Check sheet for the modelled part. Datum: model origin and axes. Units: mm. A direction names the side the tool comes from. Round coordinates to 2 decimals unless told otherwise and drop trailing zeros. Loops run counter-clockwise (first coordinate to the right, second up) from the corner with the lowest first, then second, coordinate; pieces in that order, holes last. Notation, with made-up numbers: (17.5, -1) -> (54.5, -1) arc R23 cw to (54.5, 18) -> close; hole circle Ø5 at (15, 34). An arc over 180 degrees is marked (long way). One line per question, with ' | ' between items.
```python
from build123d import *

# Parameters (mm, degrees)
F1_DEPTH  = 125
F2_R      = 1.85
F3_DEPTH  = 4
F5_DEPTH  = 3
F7_R      = 6
F8_DEPTH  = 25
F10_R     = 6
F11_DEPTH = 25


with BuildPart() as f1:
    # F0 (on Front) → F1 (new body)
    with BuildSketch(Plane.XZ):
        Polygon((27.4241377865, 47.5), (-27.4241377865, 47.5), (-23.9600361714, 41.5), (23.9600361714, 41.5), align=None)
    extrude(amount=F1_DEPTH)

    # F2 (on face) → F3 (cut)
    with BuildSketch(Plane(origin=(0, 0, 41.5), x_dir=(1, 0, 0), z_dir=(0, 0, -1))):
        with BuildLine():
            ThreePointArc((-13.8300180857, 120), (-11.9800180857, 118.15), (-10.1300180857, 120))
            Line((-10.1300180857, 120), (-13.8300180857, 120))
        make_face()
        with BuildLine():
            Line((-13.8300180857, 120), (-10.1300180857, 120))
            ThreePointArc((-10.1300180857, 120), (-11.9800180857, 121.85), (-13.8300180857, 120))
        make_face()
        with Locations((11.9800180857, 120)):
            Circle(F2_R)
        with BuildLine():
            ThreePointArc((-13.8300180857, 23), (-11.9800180857, 21.15), (-10.1300180857, 23))
            Line((-10.1300180857, 23), (-13.8300180857, 23))
        make_face()
        with BuildLine():
            Line((-13.8300180857, 23), (-10.1300180857, 23))
            ThreePointArc((-10.1300180857, 23), (-11.9800180857, 24.85), (-13.8300180857, 23))
        make_face()
        with Locations((11.9800180857, 23)):
            Circle(F2_R)
    extrude(amount=-F3_DEPTH, mode=Mode.SUBTRACT)

    # F4 (on face) → F5 (join)
    with BuildSketch(Plane.XY.offset(47.5)):
        Polygon((0.5340071506, -61.535328541), (-0.4659928494, -62.1126788102), (-0.4659928494, -65.5259274643), (-0.4659928494, -66.6806280026), (-0.4659928494, -67.4806280026), (-0.4659928494, -68.635328541), (-0.4659928494, -69.3806280026), (1.5340071506, -69.3806280026), (1.5340071506, -68.635328541), (1.5340071506, -67.4806280026), (1.5340071506, -66.6806280026), (1.5340071506, -65.5259274643), (1.5340071506, -62.1126788102), align=None)
        Polygon((2.900031855, -68.2693027335), (1.5340071506, -67.4806280026), (1.5340071506, -68.635328541), (2.4000325544, -69.135328541), align=None)
        Polygon((4.132083362, -67.0259274643), (1.5340071506, -65.5259274643), (1.5340071506, -66.6806280026), (3.6320840614, -67.8919532719), align=None)
        Polygon((-0.4659928494, -68.635328541), (-0.4659928494, -67.4806280026), (-1.8520648707, -68.2808770573), (-1.3320182531, -69.135328541), align=None)
        Polygon((-0.4659928494, -66.6806280026), (-0.4659928494, -65.5259274643), (-3.0640690607, -67.0259274643), (-2.5440224431, -67.880378948), align=None)
        Polygon((-3.4219535926, -66.819303541), (-3.4219535926, -63.819303541), (-4.4219535926, -64.3966538102), (-4.4219535926, -66.819303541), align=None)
        Polygon((-5.1147739156, -66.5781745553), (-5.1147739156, -64.7966538102), (-6.1147739156, -65.3740040794), (-6.1147739156, -66.5781745553), align=None)
        Polygon((-7.1147739156, -63.6419532718), (-6.1147739156, -63.0646030026), (-7.6576161382, -62.1738426302), (-8.1576161382, -63.039868034), align=None)
        Polygon((-5.4219535926, -62.6646030026), (-4.4219535926, -62.0872527334), (-7.0200298039, -60.5872527335), (-7.5200298039, -61.4532781373), align=None)
        Polygon((-4.4219535925, -58.6740032718), (-5.4219535925, -58.0966530026), (-7.5200298039, -59.307977868), (-7.0200298039, -60.1740032718), align=None)
        Polygon((-8.1576161382, -57.7213879713), (-7.6576161382, -58.5874133751), (-6.1147739156, -57.6966530026), (-7.1147739156, -57.1193027334), align=None)
        Polygon((-6.1147739156, -54.18308145), (-6.1147739156, -55.3872519259), (-5.1147739156, -55.964602195), (-5.1147739156, -54.18308145), align=None)
        Polygon((-4.4219535926, -53.9419524643), (-4.4219535926, -56.3646021951), (-3.4219535925, -56.9419524642), (-3.4219535926, -53.9419524643), align=None)
        Polygon((-3.0640690607, -53.735328541), (-0.4659928494, -55.235328541), (-0.4659928494, -54.0806280026), (-2.5440224431, -52.8808770573), align=None)
        Polygon((-1.8520648707, -52.480378948), (-0.4659928494, -53.2806280026), (-0.4659928494, -52.1259274643), (-1.3320182531, -51.6259274643), align=None)
        Polygon((1.5340071506, -52.1259274643), (1.5340071506, -53.2806280026), (2.900031855, -52.4919532718), (2.4000325544, -51.6259274643), align=None)
        Polygon((1.5340071506, -54.0806280026), (1.5340071506, -55.235328541), (4.132083362, -53.735328541), (3.6320840614, -52.8693027334), align=None)
        Polygon((4.4899678938, -53.9419524643), (4.4899678938, -56.9419524643), (5.4899678938, -56.3646021951), (5.4899678938, -53.9419524643), align=None)
        Polygon((6.1827882169, -54.18308145), (6.1827882169, -55.9646021951), (7.1827882169, -55.3872519259), (7.1827882169, -54.18308145), align=None)
        Polygon((8.1827882169, -57.1193027334), (7.1827882169, -57.6966530026), (8.7256304395, -58.5874133751), (9.2256304395, -57.7213879713), align=None)
        Polygon((6.4899678939, -58.0966530026), (5.4899678939, -58.6740032718), (8.0880441052, -60.1740032718), (8.5880441052, -59.307977868), align=None)
        Polygon((8.0880441052, -60.5872527335), (5.4899678939, -62.0872527335), (6.4899678939, -62.6646030027), (8.5880441052, -61.4532781373), align=None)
        Polygon((8.7256304395, -62.1738426302), (7.1827882169, -63.0646030027), (8.1827882169, -63.6419532719), (9.2256304395, -63.039868034), align=None)
        Polygon((7.1827882169, -65.3740040794), (6.1827882169, -64.7966538102), (6.1827882169, -66.5781745553), (7.1827882169, -66.5781745553), align=None)
        Polygon((2.5340071506, -60.3806280026), (1.5340071506, -60.9579782718), (1.5340071506, -62.1126788102), (4.4899678938, -63.819303541), (5.4899678938, -64.3966538102), (6.1827882169, -64.7966538102), (7.1827882169, -65.3740040794), (7.8282364841, -65.7466538103), (8.8282350853, -64.0146021951), (8.1827882169, -63.6419532719), (7.1827882169, -63.0646030027), (6.4899678939, -62.6646030027), (5.4899678939, -62.0872527335), align=None)
        Polygon((-0.4659928494, -60.9579782718), (-1.4659928493, -60.3806280026), (-4.4219535926, -62.0872527334), (-5.4219535926, -62.6646030026), (-6.1147739156, -63.0646030026), (-7.1147739156, -63.6419532718), (-7.7602214834, -64.0146025988), (-6.7602214834, -65.7466534064), (-6.1147739156, -65.3740040794), (-5.1147739156, -64.7966538102), (-4.4219535926, -64.3966538102), (-3.4219535926, -63.819303541), (-0.4659928494, -62.1126788102), align=None)
        Polygon((-7.1147739156, -57.1193027334), (-6.1147739156, -57.6966530026), (-5.4219535925, -58.0966530026), (-4.4219535925, -58.6740032718), (-1.4659928493, -60.3806280026), (-0.4659928494, -59.8032777334), (-0.4659928494, -58.648577195), (-3.4219535925, -56.9419524642), (-4.4219535925, -56.364602195), (-5.1147739156, -55.964602195), (-6.1147739156, -55.3872519258), (-6.7602221828, -55.014602195), (-7.760220784, -56.7466538101), align=None)
        Polygon((1.5340071506, -58.648577195), (1.5340071506, -59.8032777334), (2.5340071506, -60.3806280026), (5.4899678939, -58.6740032718), (6.4899678939, -58.0966530026), (7.1827882169, -57.6966530026), (8.1827882169, -57.1193027334), (8.8282357847, -56.7466534064), (7.8282357847, -55.0146025988), (7.1827882169, -55.3872519259), (6.1827882169, -55.9646021951), (5.4899678938, -56.3646021951), (4.4899678938, -56.9419524643), align=None)
        Polygon((-0.4659928494, -55.235328541), (-0.4659928494, -58.648577195), (0.5340071506, -59.2259274642), (1.5340071506, -58.648577195), (1.5340071506, -55.235328541), (1.5340071506, -54.0806280026), (1.5340071506, -53.2806280026), (1.5340071506, -52.1259274643), (1.5340071506, -51.3806280026), (-0.4659928494, -51.3806280026), (-0.4659928494, -52.1259274643), (-0.4659928494, -53.2806280026), (-0.4659928494, -54.0806280026), align=None)
        Polygon((5.4899678938, -64.3966538102), (4.4899678938, -63.819303541), (4.4899678938, -66.819303541), (5.4899678938, -66.819303541), align=None)
        Polygon((0.5340071506, -61.535328541), (-0.4659928494, -60.9579782718), (-0.4659928494, -62.1126788102), align=None)
        Polygon((1.5340071506, -60.9579782718), (0.5340071506, -61.535328541), (1.5340071506, -62.1126788102), align=None)
        Polygon((2.5340071506, -60.3806280026), (1.5340071506, -59.8032777334), (1.5340071506, -60.9579782718), align=None)
        Polygon((1.5340071506, -58.648577195), (0.5340071506, -59.2259274642), (1.5340071506, -59.8032777334), align=None)
        Polygon((0.5340071506, -59.2259274642), (-0.4659928494, -59.8032777334), (-0.4659928494, -60.9579782718), (0.5340071506, -61.535328541), (1.5340071506, -60.9579782718), (1.5340071506, -59.8032777334), align=None)
        Polygon((-0.4659928494, -59.8032777334), (-1.4659928493, -60.3806280026), (-0.4659928494, -60.9579782718), align=None)
        Polygon((-0.4659928494, -58.648577195), (-0.4659928494, -59.8032777334), (0.5340071506, -59.2259274642), align=None)
    extrude(amount=F5_DEPTH)

    # F7 (on face) → F8 (cut)
    with BuildSketch(Plane(origin=(-23.9600361714, 0, 41.5), x_dir=(0.8660254038, 0, 0.5), z_dir=(0.5, 0, -0.8660254038))):
        with Locations((0, 62.5)):
            Circle(F7_R)
    extrude(amount=F8_DEPTH, mode=Mode.SUBTRACT)

    # F10 (on face) → F11 (cut)
    with BuildSketch(Plane(origin=(23.9600361714, 0, 41.5), x_dir=(0.8660254038, 0, -0.5), z_dir=(0.5, 0, 0.8660254038))):
        with Locations((0, -62.5)):
            Circle(F10_R)
    extrude(amount=-F11_DEPTH, mode=Mode.SUBTRACT)


solid = f1.part
```
(1) Sectioned sample at B-B, the plane z = 43. Count the separate pieces of the cut face and the enclosed holes in it, and give its area (3 significant figures).
Answer:
separate pieces: 1 | enclosed holes: 6 | area: 6,110 mm2
(2) Scan lines: probe 1 along Z at (x, y) = (-11, -36); probe 2 along Y at (x, z) = (-6.5, 48.5); probe 3 along Y at (x, z) = (11, 42). Record each from-to range of solid material in increasing order.
Answer:
probe 1: z = 41.5 to 47.5 | probe 2: y = -65.6 to -62.84, -62.04 to -60.89, -59.87 to -58.72, -57.92 to -55.16 | probe 3: y = -125 to -121.57, -118.43 to -24.57, -21.43 to 0
(3) Mould release check, pull along Y, two halves, no side actions. Record for faces 5 (the face through (0, -125, 45)), 6 (the face through (6.807, -61.327, 48.979)), 7 (the face through (0, -60, 50.5)): +Y half, -Y half, draft (parallel to the pull), parting line (faces both ways), or undercut.
Answer:
face 5: -Y half | face 6: undercut | face 7: draft
(4) Set-up check for faces 1 (the face through (11.739, -121.834, 43.472)), 2 (the face through (25.67, -61.62, 44.46)), 3 (the face through (-3.422, -65, 49)), 4 (the face through (-1.747, -66.265, 48.979)): record each of +Z, -Z, +X, -X, +Y, -Y from which the full face is reachable in a straight line by a thin tool's end or side.
Answer:
face 1: -Z | face 2: -Z, +X, +Y, -Y | face 3: +Z, -Y | face 4: +Z
(5) Go/stop test with flat-tipped pins: pin 1 (1.4 mm diameter, centred on y = -65.5, z = 49, fed in from +X); pin 2 (1.1 mm diameter, centred on x = 6.5, z = 49.5, fed in from -Y); pin 3 (4 mm diameter, centred on y = -60.5, z = 47, fed in from -X). Record where each tip stops, or that it passes through.
Answer:
pin 1: stops at x = 8.37 | pin 2: stops at y = -66.58 | pin 3: stops at x = -27.42
(6) Sectioned sample at C-C, the plane y = -40. Record the cut outline in (x, z).
Answer:
outline: (-27.42, 47.5) -> (-23.96, 41.5) -> (23.96, 41.5) -> (27.42, 47.5) -> close
(7) Sectioned sample at A-A, the plane y = -120. Record the cut outline in (x, z).
Answer:
outline: (-27.42, 47.5) -> (-23.96, 41.5) -> (-13.83, 41.5) -> (-13.83, 45.5) -> (-10.13, 45.5) -> (-10.13, 41.5) -> (10.13, 41.5) -> (10.13, 45.5) -> (13.83, 45.5) -> (13.83, 41.5) -> (23.96, 41.5) -> (27.42, 47.5) -> close
